Autodesk Inventor part; units mm, degrees
ref_plane "YZ Plane" through (0, 0, 0) normal (1, 0, 0) x (0, 1, 0)
ref_plane "XZ Plane" through (0, 0, 0) normal (0, 1, 0) x (-1, 0, 0)
ref_plane "XY Plane" through (0, 0, 0) normal (0, 0, 1) x (1, 0, 0)
sketch "Sketch1" plane through (0, 0, 0) normal (0, 1, 0) x (-1, 0, 0)
  line L0 (0, 0) -> (49.8, 0)
  line L1 (49.8, 0) -> (49.8, -49.8)
  line L2 (49.8, -49.8) -> (0, -49.8)
  line L3 (0, -49.8) -> (0, 0)
  line L4 (7.8, -7.8) -> (42, -7.8)
  line L5 (42, -7.8) -> (42, -42)
  line L6 (42, -42) -> (7.8, -42)
  line L7 (7.8, -42) -> (7.8, -7.8)
  dimension "d0" = 49.8
  dimension "d1" = 49.8
  dimension "d2" = 7.8
extrude "Extrusion1" add sketch "Sketch1" along normal blind 8
sketch "Sketch3" plane through (0, 0, 0) normal (0, -1, 0) x (1, 0, 0)
  line L0 (-49.8, 0) -> (0, 0)
  line L1 (-49.8, -49.8) -> (-49.8, 0)
  line L2 (0, 0) -> (-49.8, 0)
  line L3 (-49.8, 0) -> (-49.8, -10.23)
  line L4 (-49.8, -10.23) -> (0, -10.23)
  line L5 (0, -10.23) -> (0, 0)
  line L6 (-7.8, -42) -> (-7.8, -7.8)
  line L7 (0, -49.8) -> (-7.8, -49.8)
  line L8 (-7.8, -49.8) -> (-7.8, -42)
  line L9 (-7.8, -42) -> (0, -42)
  line L10 (0, -42) -> (0, -49.8)
  line L11 (0, -49.8) -> (-49.8, -49.8)
  line L12 (-42, -7.8) -> (-42, -42)
  line L13 (-49.8, -49.8) -> (-42, -49.8)
  line L14 (-42, -49.8) -> (-42, -42)
  line L15 (-42, -42) -> (-49.8, -42)
  line L16 (-49.8, -42) -> (-49.8, -49.8)
  dimension "d6" = 10.23
extrude "Extrusion2" add sketch "Sketch3" against normal blind 97 contours L0 L5 L4 L1 | L15 L14 L11 L1 | L9 L10 L7 L8
sketch "Sketch4" plane through (-49.8, 0, 0) normal (0, 0, 1) x (1, 0, 0)
  line L0 (23.45, 81) -> (26.35, 81)
  line L1 (26.35, 81) -> (26.35, 11)
  line L2 (26.35, 11) -> (23.45, 11)
  line L3 (23.45, 11) -> (23.45, 81)
  line L4 (49.8, 0) -> (49.8, 97)
  line L5 (0, 0) -> (49.8, 0)
  circle A0 centre (24.9, 81) radius 1.45
  circle A1 centre (24.9, 11) radius 1.45
  circle A2 centre (16.4, 87) radius 1.45
  circle A3 centre (33.4, 87) radius 1.45
  line L6 (0, 97) -> (49.8, 97)
  circle A4 centre (16.4, 79) radius 1.45
  circle A5 centre (33.4, 79) radius 1.45
  circle A6 centre (16.4, 71) radius 1.45
  circle A7 centre (33.4, 71) radius 1.45
  circle A8 centre (16.4, 63) radius 1.45
  circle A9 centre (33.4, 63) radius 1.45
  circle A10 centre (16.4, 55) radius 1.45
  circle A11 centre (33.4, 55) radius 1.45
  circle A12 centre (16.4, 47) radius 1.45
  circle A13 centre (33.4, 47) radius 1.45
  circle A14 centre (16.4, 39) radius 1.45
  circle A15 centre (33.4, 39) radius 1.45
  circle A16 centre (16.4, 31) radius 1.45
  circle A17 centre (33.4, 31) radius 1.45
  circle A18 centre (16.4, 23) radius 1.45
  circle A19 centre (33.4, 23) radius 1.45
  circle A20 centre (16.4, 15) radius 1.45
  circle A21 centre (33.4, 15) radius 1.45
  point P0 (32.35, 97)
  point P1 (34.45, 97)
  dimension "d9" = 2.9
  dimension "d10" = 70
  dimension "d11" = 23.45
  dimension "d12" = 11
  dimension "d15" = 2.9
  dimension "d16" = 7.05
  dimension "d17" = 2.9
  dimension "d18" = 7.05
  dimension "d19" = 10
  dimension "d20" = 10
  dimension "d23" = 8
  dimension "d52" = 8
extrude "Extrusion3" cut sketch "Sketch4" against normal through all
sketch "Sketch5" plane through (0, 97, 0) normal (0, 1, 0) x (1, 0, 0)
  circle A0 centre (-45.9, 45.9) radius 1.4
  circle A1 centre (-3.9, 45.9) radius 1.4
  line L0 (-49.8, 49.8) -> (-49.8, 0)
  line L1 (-49.8, 24.9) -> (-42, 24.9)
  line L2 (-42, 10.23) -> (-42, 42)
  circle A2 centre (-45.9, 3.9) radius 1.4
  circle A3 centre (-3.9, 3.9) radius 1.4
  point P0 (0, 0)
  dimension "d28" = 2.8
  dimension "d29" = 2.8
extrude "Extrusion4" cut sketch "Sketch5" against normal blind 20
sketch "Sketch6" plane through (0, 0, 0) normal (0, -1, 0) x (1, 0, 0)
  line L0 (-49.8, 0) -> (0, 0)
  circle A0 centre (-24.9, -3.7) radius 1.4
  line L1 (-49.8, -49.8) -> (-49.8, 0)
  dimension "d37" = 2.8
  dimension "d38" = 3.7
  dimension "d39" = 24.9
extrude "Extrusion5" cut sketch "Sketch6" against normal blind 10
fillet "Fillet1" radius 2 4 edges at (0, 48.5, 0) (0, 48.5, -49.8) (-49.8, 48.5, -49.8) (-49.8, 48.5, 0)
sketch "Sketch7" plane through (0, 97, 0) normal (0, 1, 0) x (1, 0, 0)
  circle A0 centre (-24.9, 3.7) radius 1.4
  circle A1 centre (-24.9, 3.7) radius 1.4
  point P0 (0, 0)
extrude "Extrusion6" cut sketch "Sketch7" against normal blind 10
ref_plane "Arbeitsebene1" through (-24.9, 8, -10.23) normal (-1, 0, 0) x (0, 0, 1)
ref_plane "Arbeitsebene2" through (-47.8, 0, -24.9) normal (0, 0, 1) x (1, 0, 0)
sketch "Skizze8" plane through (0, 0, 0) normal (0, -1, 0) x (1, 0, 0)
  line L0 (-49.9, -29.9) -> (-49.9, -47.9)
  arc A0 (-49.9, -47.9) -> (-47.9, -49.9) centre (-47.9, -47.9) ccw
  line L1 (-30.0511, -49.9) -> (-47.9, -49.9)
  line L2 (-30.0511, -49.9) -> (-30.0509, -49.1742)
  arc A1 (-30.0509, -49.1742) -> (-30.2806, -48.8498) centre (-30.3999, -49.1778) ccw
  arc A2 (-31.9947, -46.7407) -> (-30.2806, -48.8498) centre (-29.84, -46.7407) ccw
  line L3 (-31.9947, -46.7407) -> (-31.9947, -46.6009)
  arc A3 (-29.8434, -44.4498) -> (-31.9947, -46.6009) centre (-29.8435, -46.6009) ccw
  line L4 (-29.8434, -44.4498) -> (-19.9598, -44.4503)
  arc A4 (-17.81, -46.6004) -> (-19.9598, -44.4503) centre (-19.96, -46.6003) ccw
  line L5 (-17.81, -46.6004) -> (-17.81, -46.7408)
  arc A5 (-19.52, -48.8451) -> (-17.81, -46.7408) centre (-19.9599, -46.7406) ccw
  arc A6 (-19.52, -48.8451) -> (-19.7498, -49.1739) centre (-19.3996, -49.1739) ccw
  line L6 (-19.7498, -49.1739) -> (-19.7495, -49.9)
  line L7 (-1.9, -49.9) -> (-19.7495, -49.9)
  arc A7 (-1.9, -49.9) -> (0.1, -47.9) centre (-1.9, -47.9) ccw
  line L8 (0.1, -47.9) -> (0.1, -30.0511)
  line L9 (0.1, -30.0511) -> (-0.6258, -30.0509)
  arc A8 (-0.6258, -30.0509) -> (-0.9502, -30.2806) centre (-0.6222, -30.3999) ccw
  arc A9 (-3.0593, -31.9947) -> (-0.9502, -30.2806) centre (-3.0593, -29.84) ccw
  line L10 (-3.0593, -31.9947) -> (-3.1991, -31.9947)
  arc A10 (-5.3502, -29.8434) -> (-3.1991, -31.9947) centre (-3.1991, -29.8435) ccw
  line L11 (-5.3502, -29.8434) -> (-5.3497, -19.9598)
  arc A11 (-3.1996, -17.81) -> (-5.3497, -19.9598) centre (-3.1997, -19.96) ccw
  line L12 (-3.1996, -17.81) -> (-3.0592, -17.81)
  arc A12 (-0.9549, -19.52) -> (-3.0592, -17.81) centre (-3.0594, -19.9599) ccw
  arc A13 (-0.9549, -19.52) -> (-0.6261, -19.7498) centre (-0.6261, -19.3996) ccw
  line L13 (-0.6261, -19.7498) -> (0.1, -19.7495)
  line L14 (0.1, -19.7495) -> (0.1, -1.9)
  arc A14 (0.1, -1.9) -> (-1.9, 0.1) centre (-1.9, -1.9) ccw
  line L15 (-19.9, 0.1) -> (-1.9, 0.1)
  line L16 (-19.9, 0.1) -> (-19.9, 0.9263)
  arc A15 (-19.56, 1.4) -> (-19.9, 0.9263) centre (-19.4, 0.9263) ccw
  arc A16 (-19.56, 1.4) -> (-17.96, 3.3596) centre (-19.96, 3.3596) ccw
  line L17 (-17.96, 3.3596) -> (-17.96, 3.5)
  arc A17 (-17.96, 3.5) -> (-19.96, 5.5) centre (-19.96, 3.5) ccw
  line L18 (-19.96, 5.5) -> (-29.84, 5.5)
  arc A18 (-29.84, 5.5) -> (-31.84, 3.5) centre (-29.84, 3.5) ccw
  line L19 (-31.84, 3.5) -> (-31.84, 3.3596)
  arc A19 (-31.84, 3.3596) -> (-30.24, 1.4) centre (-29.84, 3.3596) ccw
  arc A20 (-29.9, 0.9263) -> (-30.24, 1.4) centre (-30.4, 0.9263) ccw
  line L20 (-29.9, 0.9263) -> (-29.9, 0.1)
  line L21 (-47.9, 0.1) -> (-29.9, 0.1)
  arc A21 (-47.9, 0.1) -> (-49.9, -1.9) centre (-47.9, -1.9) ccw
  line L22 (-49.9, -1.9) -> (-49.9, -19.9)
  line L23 (-49.9, -19.9) -> (-50.7263, -19.9)
  arc A22 (-51.2, -19.56) -> (-50.7263, -19.9) centre (-50.7263, -19.4) ccw
  arc A23 (-51.2, -19.56) -> (-53.1596, -17.96) centre (-53.1596, -19.96) ccw
  line L24 (-53.1596, -17.96) -> (-53.3, -17.96)
  arc A24 (-53.3, -17.96) -> (-55.3, -19.96) centre (-53.3, -19.96) ccw
  line L25 (-55.3, -19.96) -> (-55.3, -29.84)
  arc A25 (-55.3, -29.84) -> (-53.3, -31.84) centre (-53.3, -29.84) ccw
  line L26 (-53.3, -31.84) -> (-53.1596, -31.84)
  arc A26 (-53.1596, -31.84) -> (-51.2, -30.24) centre (-53.1596, -29.84) ccw
  arc A27 (-50.7263, -29.9) -> (-51.2, -30.24) centre (-50.7263, -30.4) ccw
  line L27 (-50.7263, -29.9) -> (-49.9, -29.9)
  arc A28 (-49.9, -26.2329) -> (-49.9, -23.7671) centre (-46.2, -25) ccw
  line L28 (-49.9, -26.2329) -> (-49.9, -23.7671)
  circle A29 centre (-25, -3.6) radius 3.9
  line L29 (-7.6, -40.2) -> (-7.6, -9.6)
  arc A30 (-9.6, -42.2) -> (-7.6, -40.2) centre (-9.6, -40.2) ccw
  line L30 (-9.6, -42.2) -> (-40.2, -42.2)
  arc A31 (-42.2, -40.2) -> (-40.2, -42.2) centre (-40.2, -40.2) ccw
  line L31 (-42.2, -9.6) -> (-42.2, -40.2)
  arc A32 (-40.2, -7.6) -> (-42.2, -9.6) centre (-40.2, -9.6) ccw
  line L32 (-40.2, -7.6) -> (-9.6, -7.6)
  arc A33 (-7.6, -9.6) -> (-9.6, -7.6) centre (-9.6, -9.6) ccw
  circle A34 centre (-44.8, -5) radius 2.4
  circle A35 centre (-39.35, -4.35) radius 2.45
  circle A36 centre (-45.45, -10.45) radius 2.45
  circle A37 centre (-4.35, -10.45) radius 2.45
  circle A38 centre (-10.45, -4.35) radius 2.45
  circle A39 centre (-5, -5) radius 2.4
  circle A40 centre (-45.45, -39.35) radius 2.45
  circle A41 centre (-39.35, -45.45) radius 2.45
  circle A42 centre (-44.8, -44.8) radius 2.4
  circle A43 centre (-4.35, -39.35) radius 2.45
  circle A44 centre (-10.45, -45.45) radius 2.45
  circle A45 centre (-5, -44.8) radius 2.4
  point P0 (0, 0)
hole "Bohrung1" at (-45.45, 0, -39.35) at (-45.45, 0, -10.45) at (-39.35, 0, -4.35) at (-10.45, 0, -4.35) at (-4.35, 0, -10.45) at (-4.35, 0, -39.35) at (-10.45, 0, -45.45) at (-39.35, 0, -45.45) direction (0, 1, 0) diameter 4.6 end through all
properties part number "00_Linear_Stage_NEMA11_Mount"
Work out the finished part from the listing and answer in its coordinate system (mm). A direction names the side the tool comes from. Give positions to 0.01 mm unless a question says otherwise; leave off trailing zeros. Write each loop counter-clockwise with the first axis right and the second up, starting at its lowest first coordinate (ties: lowest second). Pieces come first, ordered by that corner, then holes. Notation, with made-up numbers: (0.5, 73.5) - (13.5, 73.5) arc R19 ccw to (13.5, 89.5) - close; hole circle Ø2 at (82.5, -32.75). An arc over 180 degrees is marked (long way). Use one line per item in the form item = value.
1. Each of these flat-tipped pins is pushed along its axis until it touches: pin 1 Ø3.5 at (x, y) = (-33.4, 15) entering from +Z; pin 2 Ø4 at (x, z) = (-20, -45.5) entering from +Y; pin 3 Ø4 at (x, y) = (-16.4, 15) entering from -Z. Where does it stop, or does it pass through?
Filled in:
pin_1 = 0
pin_2 = 8
pin_3 = -10.23
2. A cutting plane is placed at C-C (y = 50.5). Write down the section's boundary in (x, z).
Filled in:
outline = (-49.8, -47.8) arc R2 ccw to (-47.8, -49.8) - (-42, -49.8) - (-42, -42) - (-49.8, -42) - close; (-49.8, -10.23) - (-47.74, -10.23) arc R2.3 cw to (-43.16, -10.23) - (-26.35, -10.23) - (-26.35, 0) - (-47.8, 0) arc R2 ccw to (-49.8, -2) - close; (-23.45, -10.23) - (-6.64, -10.23) arc R2.3 cw to (-2.06, -10.23) - (0, -10.23) - (0, -2) arc R2 ccw to (-2, 0) - (-23.45, 0) - close; (-7.8, -49.8) - (-2, -49.8) arc R2 ccw to (0, -47.8) - (0, -42) - (-7.8, -42) - close; hole circle Ø4.6 at (-39.35, -4.35); hole circle Ø4.6 at (-10.45, -4.35)
3. For faces 4 (the face through (-16.714, 69.584, -5.043)), 5 (the face through (-46, 8, -26)), 6 (the face through (-49.8, 37, -9)), 7 (the face through (-25, 8, -46)), 8 (the face through (-25, 87, -4)), determine the directions among +Z, -Z, +X, -X, +Y, -Y from which every point of the face is accessible in a straight line to the end or side of a thin tool.
Filled in:
face_4 = +Z, -Z
face_5 = +X, -X, +Y
face_6 = +Z, -Z, -X, +Y, -Y
face_7 = -Z, +Y
face_8 = +Y
4. Consider L1, parallel to Z at x = -48, y = 29; L2, parallel to Z at x = -43.5, y = 4.5; L3, parallel to X at y = 52, z = -44.5. Determine where each line is inside the solid, lowest interval first.
Filled in:
L1 = -49.79 to -42, -10.23 to -0.01
L2 = -49.8 to -40.57, -38.13 to -11.67, -9.23 to 0
L3 = -49.8 to -42, -7.8 to 0
5. A cutting plane is placed at D-D (z = -32). Write down the section's boundary in (x, y).
Filled in:
outline = (-49.8, 0) - (-42, 0) - (-42, 8) - (-49.8, 8) - close; (-7.8, 0) - (0, 0) - (0, 8) - (-7.8, 8) - close
6. Determine the mould class of faces 1 (the face through (-17.55, 54.12, -5.04)), 2 (the face through (-25, 97, -6)), 3 (the face through (-0.57, 49.18, -49.2)) for opening direction X: released by +X, released by -X, zero draft, split by the parting line, or undercut.
Filled in:
face_1 = undercut
face_2 = zero draft
face_3 = released by +X
7. A cutting plane is placed at B-B (x = -39.35). Write down the section's boundary in (y, z).
Filled in:
outline = (0, -49.8) - (8, -49.8) - (8, -47.75) - (0, -47.75) - close; (0, -43.15) - (8, -43.15) - (8, -42) - (0, -42) - close; (0, -10.23) - (97, -10.23) - (97, -6.65) - (0, -6.65) - close; (0, -2.05) - (97, -2.05) - (97, 0) - (0, 0) - close
8. A cutting plane is placed at A-A (y = 71). State how many separate pieces and enclosed holes the cut face has, and give its area (3 significant figures).
Filled in:
separate_pieces = 6
enclosed_holes = 2
area = 491 mm^2
